For this review, take the finished solid that the model builds, in its own axes (mm). Coordinates: 2 decimals unless noted, no trailing zeros. Write each loop counter-clockwise with the first axis right and the second up, starting at its lowest first coordinate (ties: lowest second). Pieces come first, ordered by that corner, then holes.
1) Mouldability with a two-part tool opening along Z and no side actions: class faces 1 (the face through (344.317, 1.61, -58.265)), 2 (the face through (-23.79, 1.61, -107.15)), 3 (the face through (414.85, 1.61, -3.01)) as pulls with the +Z half, pulls with the -Z half, needs draft (parallel to the pull), parting line crosses it, or undercut.
2) We need section A-A on x = 228. Write out the cut boundary in (y, z) (3 decimals), then the cut area to 3 significant figures.
3) We need section B-B on y = 0.7. Give the number of separate pieces and of enclosed holes in the cut face, then the cut area to 3 significant figures.
4) Insertion check: P1, Ø4.5, axis at x = 147.45, z = -10, coming from the +Y side (3 decimals). The pin has a flat end and moves straight along its axis. Give the tip position at first contact, or say it passes through.
5) To check wall thickness, follow line 1 along Z through (x, y) = (87, 1.25); line 2 along Z through (x, y) = (27.5, 0.2); line 3 along Z through (x, y) = (348.5, 2.3). State the ranges of each line that lie inside material, in increasing order.
from build123d import *

# Parameters (mm, degrees)
SKETCH1_R           = 2
SKETCH1_R_2         = 6
SKETCH1_R_3         = 1.5
BOSS_EXTRUDE1_DEPTH = 3.175
FILLET1_R           = 10
CUT_EXTRUDE1_DEPTH  = 10


with BuildPart() as part:
    # Sketch1 → Boss-Extrude1 (new body)
    with BuildSketch(Plane(origin=(0, 0, 0), x_dir=(1, 0, 0), z_dir=(0, 1, 0))):
        Polygon((417.700422465, 110), (-26.799577535, 110), (-26.799577535, 0), (417.700422465, 0), (417.700422465, 17.22815868), align=None)
        with Locations(Location((147.450422465, 10, 0), (0, 0, 270))):
            Circle(SKETCH1_R, mode=Mode.SUBTRACT)
        with Locations(Location((23.200422465, 40, 0), (0, 0, 270))):
            Circle(SKETCH1_R, mode=Mode.SUBTRACT)
        with Locations(Location((282.700422465, 17.22815868, 0), (0, 0, 270))):
            Circle(SKETCH1_R_2, mode=Mode.SUBTRACT)
        with Locations(Location((367.700422465, 40, 0), (0, 0, 270))):
            Circle(SKETCH1_R, mode=Mode.SUBTRACT)
        with Locations(Location((-16.799577535, 85, 0), (0, 0, 270))):
            Circle(SKETCH1_R, mode=Mode.SUBTRACT)
        with Locations(Location((-19.299577535, 102.5, 0), (0, 0, 270))):
            Circle(SKETCH1_R_3, mode=Mode.SUBTRACT)
        with Locations(Location((88.075422465, 102.5, 0), (0, 0, 270))):
            Circle(SKETCH1_R_3, mode=Mode.SUBTRACT)
        with Locations(Location((147.450422465, 85, 0), (0, 0, 270))):
            Circle(SKETCH1_R, mode=Mode.SUBTRACT)
        with Locations(Location((279.700422465, 85, 0), (0, 0, 270))):
            Circle(SKETCH1_R, mode=Mode.SUBTRACT)
        with Locations(Location((195.450422465, 102.5, 0), (0, 0, 270))):
            Circle(SKETCH1_R_3, mode=Mode.SUBTRACT)
        with Locations(Location((302.825422465, 102.5, 0), (0, 0, 270))):
            Circle(SKETCH1_R_3, mode=Mode.SUBTRACT)
        with Locations(Location((407.700422465, 85, 0), (0, 0, 270))):
            Circle(SKETCH1_R, mode=Mode.SUBTRACT)
        with Locations(Location((410.200422465, 102.5, 0), (0, 0, 270))):
            Circle(SKETCH1_R_3, mode=Mode.SUBTRACT)
    extrude(amount=BOSS_EXTRUDE1_DEPTH)

    # Fillet1
    fillet1_edges = [part.edges().sort_by_distance(p)[0] for p in [
        (-26.799577535, 1.5875, -110),
        (417.700422465, 1.5875, -110),
        (417.700422465, 1.5875, 0),
        (-26.799577535, 1.5875, 0),
    ]]
    fillet(fillet1_edges, radius=FILLET1_R)

    # Sketch2 → Cut-Extrude1 (cut)
    with BuildSketch(Plane(origin=(0, 3.175, 0), x_dir=(1, 0, 0), z_dir=(0, 1, 0))):
        with BuildLine():
            Line((63.988295206, 24.860334116), (26.456586442, 33.922316112))
            ThreePointArc((26.456586442, 33.922316112), (24.273585164, 33.959016834), (22.283065126, 33.061981996))
            Line((22.283065126, 33.061981996), (10.200422465, 24))
            ThreePointArc((10.200422465, 24), (8.457005975, 18.41886117), (13.200422465, 15))
            Line((13.200422465, 15), (62.81477389, 15))
            ThreePointArc((62.81477389, 15), (67.779734645, 19.409098393), (63.988295206, 24.860334116))
        make_face()
        with BuildLine():
            Line((1.731814293, 71.678180806), (21.183909441, 49.794573764))
            ThreePointArc((21.183909441, 49.794573764), (25.478109933, 49.737152551), (29.35222616, 47.883863983))
            Line((29.35222616, 47.883863983), (83.514557274, 67.5))
            Line((83.514557274, 67.5), (91.361350439, 70.2886824))
            ThreePointArc((91.361350439, 70.2886824), (94.61428981, 75.849532813), (89.686988926, 80))
            Line((89.686988926, 80), (5.468860886, 80))
            ThreePointArc((5.468860886, 80), (0.907660607, 77.048280258), (1.731814293, 71.678180806))
        make_face()
        with BuildLine():
            ThreePointArc((13.203172612, 39.765489068), (13.250707237, 41.001582191), (13.450490987, 42.222349247))
            ThreePointArc((13.450490987, 42.222349247), (13.034220935, 43.599450655), (12.243072673, 44.801021905))
            Line((12.243072673, 44.801021905), (-3.062530941, 62.019825971))
            ThreePointArc((-3.062530941, 62.019825971), (-8.576480322, 63.371615284), (-11.799577535, 58.698006777))
            Line((-11.799577535, 58.698006777), (-11.799577535, 30))
            ThreePointArc((-11.799577535, 30), (-9.035645512, 25.527864045), (-3.799577535, 26))
            Line((-3.799577535, 26), (11.506026079, 37.479202711))
            ThreePointArc((11.506026079, 37.479202711), (12.520785414, 38.498983342), (13.203172612, 39.765489068))
        make_face()
        with BuildLine():
            Line((47.554716749, 39.2633668), (136.276901149, 17.841511412))
            ThreePointArc((136.276901149, 17.841511412), (140.543349349, 18.773257577), (142.450422465, 22.701845528))
            Line((142.450422465, 22.701845528), (142.450422465, 70.404600889))
            ThreePointArc((142.450422465, 70.404600889), (140.32155553, 74.498082894), (135.747784496, 75.105773503))
            Line((135.747784496, 75.105773503), (47.343070087, 43.087969492))
            ThreePointArc((47.343070087, 43.087969492), (46.027180577, 41.096993104), (47.554716749, 39.2633668))
        make_face()
        with BuildLine():
            Line((152.450422465, 67.944146827), (152.450422465, 27.234106769))
            ThreePointArc((152.450422465, 27.234106769), (154.931598866, 22.91490225), (159.912633536, 22.882381061))
            Line((159.912633536, 22.882381061), (197.668168627, 44.244503287))
            ThreePointArc((197.668168627, 44.244503287), (200.204889799, 48.699555799), (197.486244065, 53.045981061))
            Line((197.486244065, 53.045981061), (159.730708974, 72.393898891))
            ThreePointArc((159.730708974, 72.393898891), (154.842878846, 72.210376576), (152.450422465, 67.944146827))
        make_face()
        with BuildLine():
            Line((274.700422465, 34.284011853), (274.700422465, 67.765893231))
            ThreePointArc((274.700422465, 67.765893231), (272.219246064, 72.08509775), (267.238211394, 72.117618939))
            Line((267.238211394, 72.117618939), (236.186256017, 54.548389301))
            ThreePointArc((236.186256017, 54.548389301), (233.649534845, 50.093336789), (236.368180579, 45.746911528))
            Line((236.368180579, 45.746911528), (267.420135956, 29.834259789))
            ThreePointArc((267.420135956, 29.834259789), (272.307966085, 30.017782104), (274.700422465, 34.284011853))
        make_face()
        with BuildLine():
            Line((284.700422465, 68.076898184), (284.700422465, 33.714803321))
            ThreePointArc((284.700422465, 33.714803321), (290.246819989, 30.85104203), (294.408739409, 26.198937028))
            Line((294.408739409, 26.198937028), (340.058508189, 38.011769879))
            ThreePointArc((340.058508189, 38.011769879), (343.775835313, 42.304727092), (341.082359043, 47.304045862))
            Line((341.082359043, 47.304045862), (301.204849524, 67.695954138))
            Line((301.204849524, 67.695954138), (292.020165923, 72.506208546))
            ThreePointArc((292.020165923, 72.506208546), (287.111862758, 72.354673148), (284.700422465, 68.076898184))
        make_face()
        with BuildLine():
            Line((320.393543744, 70.570564095), (326.257240647, 67.5))
            Line((326.257240647, 67.5), (362.890344157, 48.767162978))
            ThreePointArc((362.890344157, 48.767162978), (366.212170141, 49.888635144), (369.716935489, 49.794573764))
            Line((369.716935489, 49.794573764), (389.169030638, 71.678180806))
            ThreePointArc((389.169030638, 71.678180806), (389.993184323, 77.048280258), (385.431984044, 80))
            Line((385.431984044, 80), (322.713047476, 80))
            ThreePointArc((322.713047476, 80), (317.857783347, 76.194324176), (320.393543744, 70.570564095))
        make_face()
        with BuildLine():
            Line((379.559027243, 37.88827322), (390.700422465, 29))
            Line((390.700422465, 29), (393.166651981, 27.150327863))
            ThreePointArc((393.166651981, 27.150327863), (398.402719958, 26.678191908), (401.166651981, 31.150327863))
            Line((401.166651981, 31.150327863), (401.166651981, 57.012678354))
            ThreePointArc((401.166651981, 57.012678354), (397.901307442, 61.70213146), (392.370263808, 60.266512529))
            Line((392.370263808, 60.266512529), (391.437469059, 59.178180806))
            Line((391.437469059, 59.178180806), (378.940138766, 45.118684227))
            ThreePointArc((378.940138766, 45.118684227), (377.695401669, 41.370448261), (379.559027243, 37.88827322))
        make_face()
        with BuildLine():
            Line((364.296086649, 33.954363295), (329.076499674, 24.840558227))
            ThreePointArc((329.076499674, 24.840558227), (325.369116008, 19.368648725), (330.329095399, 15))
            Line((330.329095399, 15), (377.700422465, 15))
            ThreePointArc((377.700422465, 15), (382.443838955, 18.41886117), (380.700422465, 24))
            Line((380.700422465, 24), (368.548682375, 33.113805068))
            ThreePointArc((368.548682375, 33.113805068), (366.518213167, 34.018905479), (364.296086649, 33.954363295))
        make_face()
        with BuildLine():
            Line((185.278283157, 15), (251.008650991, 15))
            ThreePointArc((251.008650991, 15), (255.869142752, 18.82713179), (253.2889375, 24.449752065))
            Line((253.2889375, 24.449752065), (218.797900418, 42.124769774))
            ThreePointArc((218.797900418, 42.124769774), (216.414300992, 42.67395024), (214.055427015, 42.026757098))
            Line((214.055427015, 42.026757098), (182.816096263, 24.351739388))
            ThreePointArc((182.816096263, 24.351739388), (180.443063568, 18.726951874), (185.278283157, 15))
        make_face()
        with BuildLine():
            Line((241.872561773, 80), (190.247225864, 80))
            ThreePointArc((190.247225864, 80), (185.386734103, 76.17286821), (187.966939355, 70.550247935))
            Line((187.966939355, 70.550247935), (215.056569824, 56.668099447))
            ThreePointArc((215.056569824, 56.668099447), (217.44016925, 56.118918981), (219.799043227, 56.766112124))
            Line((219.799043227, 56.766112124), (244.334748667, 70.648260612))
            ThreePointArc((244.334748667, 70.648260612), (246.707781362, 76.273048126), (241.872561773, 80))
        make_face()
    extrude(amount=-CUT_EXTRUDE1_DEPTH, mode=Mode.SUBTRACT)


solid = part.part
Result:
1. face 1: undercut
1. face 2: pulls with the -Z half
1. face 3: pulls with the +Z half
2. outline: (0, -110) - (3.175, -110) - (3.175, -80) - (0, -80) - close; (0, -61.406) - (3.175, -61.406) - (3.175, -37.409) - (0, -37.409) - close; (0, -15) - (3.175, -15) - (3.175, 0) - (0, 0) - close
2. area: 219 mm2
3. separate pieces: 1
3. enclosed holes: 25
3. area: 32,600 mm2
4. P1: stops at y = 3.175
5. line 1: z = -110 to -103.55, -101.45 to -80, -68.74 to -57.45, -29.74 to 0
5. line 2: z = -110 to -80, -49.03 to -33.67, -15 to 0
5. line 3: z = -110 to -80, -56.13 to -29.87, -15 to 0
